The listing builds one solid part. Answer for the finished solid, in the listing's coordinates (mm). Face numbers are marked on the shaded views. Round coordinates to 2 decimals unless told otherwise and drop trailing zeros. Loops run counter-clockwise (first coordinate to the right, second up) from the corner with the lowest first, then second, coordinate; pieces in that order, holes last. Notation, with made-up numbers: (27, 27.25) -> (84, 27.25) arc R17 cw to (84, 58.25) -> close; hole circle Ø1 at (-33.75, -20). An arc over 180 degrees is marked (long way). Use a Markdown table: item, result. Add a question column.
Q1. Section D-D on x = 5.5 is taken. Give the vertices of the cut face in (y, z) (3 decimals), then the cut area to 3 significant figures.
Q2. Section A-A on x = 0 is taken. Give the vertices of the cut face in (y, z).
Q3. Section B-B on z = 8 is taken. Give the vertices of the cut face in (x, y).
Q4. For a pull along Z with two mould halves and no side action, classify the marked faces 1, 2 and 3 as released by +Z, released by -Z, zero draft, split by the parting line, or undercut.
Q5. Section C-C on y = 6 is taken. Give the vertices of the cut face in (x, z), then the cut area to 3 significant figures.
Q6. Given pin 1 Ø4 at (x, z) = (0, 9.74) entering from +Y, flat-ended and moving along its own axis, determine where the tip first touches the part or whether it passes through.
Q7. Consider line 1 (Z direction, x = -2.5, y = 8.5); line 2 (X direction, y = 10.75, z = 7); line 3 (X direction, y = 2.5, z = 11.25). Determine where each line is inside the solid, lowest interval first.
from build123d import *

# Parameters (mm, degrees)
ESQUISSE1_R        = 3.25
BOSS_EXTRU_1_DEPTH = 17


with BuildPart() as part:
    # Esquisse1 → Boss.-Extru.1 (new body)
    with BuildSketch(Plane(origin=(0, 0, 0), x_dir=(1, 0, 0), z_dir=(0, 1, 0))):
        with BuildLine():
            Line((-14.75, 0), (14.75, 0))
            Line((14.75, 0), (14.75, -24.5))
            ThreePointArc((14.75, -24.5), (0, -21.240155954), (-14.75, -24.5))
            Line((-14.75, -24.5), (-14.75, 0))
        make_face()
        with Locations(Location((0, -9.740155954, 0), (0, 0, 270))):
            Circle(ESQUISSE1_R, mode=Mode.SUBTRACT)
    extrude(amount=BOSS_EXTRU_1_DEPTH)


solid = part.part
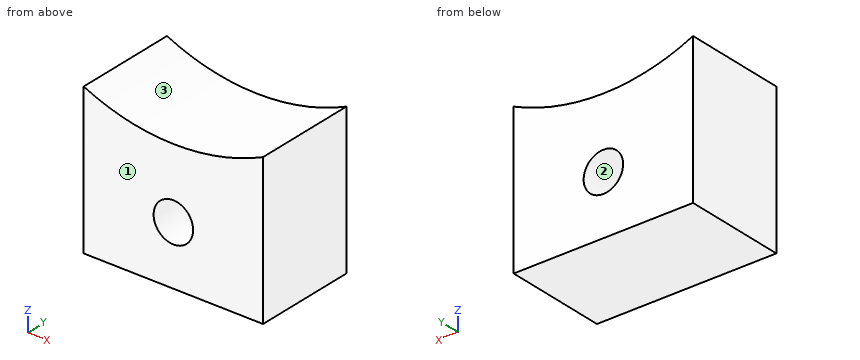
Checked values:
| question | item | result |
|---|---|---|
| 1 | outline | (0, 0) -> (17, 0) -> (17, 21.675) -> (0, 21.675) -> close |
| 1 | area | 368 mm2 |
| 2 | outline | (0, 0) -> (17, 0) -> (17, 6.49) -> (0, 6.49) -> close; (0, 12.99) -> (17, 12.99) -> (17, 21.24) -> (0, 21.24) -> close |
| 3 | outline | (-14.75, 0) -> (-2.74, 0) -> (-2.74, 17) -> (-14.75, 17) -> close; (2.74, 0) -> (14.75, 0) -> (14.75, 17) -> (2.74, 17) -> close |
| 4 | face 1 | zero draft |
| 4 | face 2 | undercut |
| 4 | face 3 | released by +Z |
| 5 | outline | (-14.75, 0) -> (14.75, 0) -> (14.75, 24.5) arc R35 cw to (-14.75, 24.5) -> close; hole circle Ø6.5 at (0, 9.74) |
| 5 | area | 625 mm2 |
| 6 | pin 1 | passes through |
| 7 | line 1 | z = 0 to 7.66, 11.82 to 21.33 |
| 7 | line 2 | x = -14.75 to -1.75, 1.75 to 14.75 |
| 7 | line 3 | x = -14.75 to -2.88, 2.88 to 14.75 |
